from build123d import *

# Parameters (mm, degrees)
BOSS_EXTRUDE1_DEPTH = 20
SKETCH2_R           = 7.5
BOSS_EXTRUDE2_DEPTH = 85
SKETCH4_R           = 6.5
BOSS_EXTRUDE3_DEPTH = 20
SKETCH5_W           = 60
SKETCH5_H           = 10
CUT_EXTRUDE1_DEPTH  = 2
FILLET1_R           = 0.5
FILLET2_R           = 0.5


with BuildPart() as part:
    # Sketch1 → Boss-Extrude1 (new body)
    with BuildSketch(Plane.XY):
        with BuildLine():
            Line((0, 0), (0, 25.5))
            ThreePointArc((0, 25.5), (2.928932188, 32.571067812), (10, 35.5))
            Line((10, 35.5), (85, 35.5))
            ThreePointArc((85, 35.5), (92.071067812, 32.571067812), (95, 25.5))
            Line((95, 25.5), (95, -25.5))
            ThreePointArc((95, -25.5), (92.071067812, -32.571067812), (85, -35.5))
            Line((85, -35.5), (10, -35.5))
            ThreePointArc((10, -35.5), (2.928932188, -32.571067812), (0, -25.5))
            Line((0, -25.5), (0, 0))
        make_face()
        with BuildLine():
            Line((10, 0), (10, 15.5))
            ThreePointArc((10, 15.5), (12.928932188, 22.571067812), (20, 25.5))
            Line((20, 25.5), (75, 25.5))
            ThreePointArc((75, 25.5), (82.071067812, 22.571067812), (85, 15.5))
            Line((85, 15.5), (85, 0))
            Line((85, 0), (85, -15.5))
            ThreePointArc((85, -15.5), (82.071067812, -22.571067812), (75, -25.5))
            Line((75, -25.5), (20, -25.5))
            ThreePointArc((20, -25.5), (12.928932188, -22.571067812), (10, -15.5))
            Line((10, -15.5), (10, 0))
        make_face(mode=Mode.SUBTRACT)
    extrude(amount=BOSS_EXTRUDE1_DEPTH)

    # Sketch2 → Boss-Extrude2 (add)
    with BuildSketch(Plane(origin=(0, 0, 0), x_dir=(0, 0, -1), z_dir=(1, 0, 0))):
        with Locations((-10, 0)):
            Circle(SKETCH2_R)
    extrude(amount=BOSS_EXTRUDE2_DEPTH)

    # Sketch4 → Boss-Extrude3 (add)
    with BuildSketch(Plane(origin=(0, 0, 0), x_dir=(0, 0, -1), z_dir=(1, 0, 0))):
        with Locations((-10, 0)):
            Circle(SKETCH4_R)
    extrude(amount=-BOSS_EXTRUDE3_DEPTH)

    # Sketch5 → Cut-Extrude1 (cut)
    with BuildSketch(Plane.XZ.offset(35.5)):
        with Locations((48, 10.5)):
            Rectangle(SKETCH5_W, SKETCH5_H)
    cut_extrude1 = extrude(amount=-CUT_EXTRUDE1_DEPTH, mode=Mode.SUBTRACT)

    # Mirror1: Cut-Extrude1 across plane
    add(cut_extrude1.mirror(Plane.ZX), mode=Mode.SUBTRACT)

    # Fillet1
    fillet1_edges = [part.edges().sort_by_distance(p)[0] for p in [
        (47.5, 35.5, 0),
        (92.071067812, 32.571067812, 0),
        (95, 0, 0),
        (92.071067812, -32.571067812, 0),
        (47.5, -35.5, 0),
        (2.928932188, -32.571067812, 0),
        (47.5, -35.5, 20),
        (92.071067812, -32.571067812, 20),
        (95, 0, 20),
        (92.071067812, 32.571067812, 20),
        (47.5, 35.5, 20),
        (2.928932188, 32.571067812, 20),
        (0, 0, 20),
        (2.928932188, -32.571067812, 20),
        (0, 0, 0),
        (2.928932188, 32.571067812, 0),
    ]]
    fillet(fillet1_edges, radius=FILLET1_R)

    # Fillet2
    fillet2_edges = [part.edges().sort_by_distance(p)[0] for p in [
        (12.928932188, -22.571067812, 0),
        (47.5, -25.5, 0),
        (82.071067812, -22.571067812, 0),
        (85, 0, 0),
        (82.071067812, 22.571067812, 0),
        (47.5, 25.5, 0),
        (12.928932188, 22.571067812, 0),
        (10, 0, 0),
        (10, 0, 20),
        (12.928932188, -22.571067812, 20),
        (47.5, -25.5, 20),
        (82.071067812, -22.571067812, 20),
        (85, 0, 20),
        (82.071067812, 22.571067812, 20),
        (47.5, 25.5, 20),
        (12.928932188, 22.571067812, 20),
    ]]
    fillet(fillet2_edges, radius=FILLET2_R)


solid = part.part
Geometry: final body of the model. Coordinates: model frame, mm. A direction names the side the tool comes from. Give positions to 0.01 mm unless a question says otherwise; leave off trailing zeros. Write each loop counter-clockwise with the first axis right and the second up, starting at its lowest first coordinate (ties: lowest second). Pieces come first, ordered by that corner, then holes.
(1) Ray query, line 1 (Y direction, x = 46, z = 2); line 2 (Y direction, x = 72, z = 14.75); line 3 (X direction, y = -16, z = 10). Return the intervals inside material, ascending.
(2) First-contact query: P1, Ø1.6, axis at y = 34, z = 10.5, coming from the -X side; P2, Ø8, axis at x = 61, y = -22.5, coming from the -Z side; P3, Ø1.6, axis at y = 34.5, z = 8, coming from the +X side; P4, Ø2, axis at x = 23.5, z = 11, coming from the -Y side. Flat tips, straight axial feed; report the tip coordinate or a pass-through.
(3) Cut plane D-D, the plane x = -10. Return loops of the section in (y, z), then the cut area to 3 significant figures.
(4) Cut plane A-A, the plane x = 25.5. Return loops of the section in (y, z), then the cut area to 3 significant figures.
(5) Cut plane C-C, the plane y = 0. Return loops of the section in (x, z), then the cut area to 3 significant figures.
(6) Cut plane B-B, the plane z = 10. Give the number of separate pieces and of enclosed holes in the cut face, then the cut area to 4 significant figures.
(7) Access query for faces 5 (the flat face through (47, 25.5, 10)), 6 (the cylindrical face through (-9.86, 1.95, 3.8)), 7 (the flat face through (48, -35.5, 4)). Directions: +Z, -Z, +X, -X, +Y, -Y. A direction counts if a zero-diameter tool reaches every point of the face in a straight line with its end or side. Return the directions, or none.
(8) Mould query, pull axis Z, two halves, no side actions, for faces 1 (the flat face through (95, 0, 10)), 2 (the flat face through (48, -33.5, 11)), 3 (the cylindrical face through (47, 5.1, 15.5)), 4 (the flat face through (48, 33.5, 11)). Classes: released by +Z, released by -Z, zero draft, split by the parting line, or undercut.
Values follow:
1. line 1: y = -35.5 to -25.5, 25.5 to 35.5
1. line 2: y = -33.5 to -25.5, -5.8 to 5.8, 25.5 to 33.5
1. line 3: x = 0 to 10.01, 84.99 to 95
2. P1: stops at x = 3.62
2. P2: stops at z = 0
2. P3: stops at x = 90.72
2. P4: stops at y = -33.5
3. outline: circle Ø13 at (0, 10)
3. area: 133 mm2
4. outline: (-35.5, 0.5) arc R0.5 ccw to (-35, 0) - (-26, 0) arc R0.5 ccw to (-25.5, 0.5) - (-25.5, 19.5) arc R0.5 ccw to (-26, 20) - (-35, 20) arc R0.5 ccw to (-35.5, 19.5) - (-35.5, 15.5) - (-33.5, 15.5) - (-33.5, 5.5) - (-35.5, 5.5) - close; circle Ø15 at (0, 10); (25.5, 0.5) arc R0.5 ccw to (26, 0) - (35, 0) arc R0.5 ccw to (35.5, 0.5) - (35.5, 5.5) - (33.5, 5.5) - (33.5, 15.5) - (35.5, 15.5) - (35.5, 19.5) arc R0.5 ccw to (35, 20) - (26, 20) arc R0.5 ccw to (25.5, 19.5) - close
4. area: 536 mm2
5. outline: (-20, 3.5) - (0, 3.5) - (0, 0.5) arc R0.5 ccw to (0.5, 0) - (9.5, 0) arc R0.5 ccw to (10, 0.5) - (10, 2.5) - (85, 2.5) - (85, 0.5) arc R0.5 ccw to (85.5, 0) - (94.5, 0) arc R0.5 ccw to (95, 0.5) - (95, 19.5) arc R0.5 ccw to (94.5, 20) - (85.5, 20) arc R0.5 ccw to (85, 19.5) - (85, 17.5) - (10, 17.5) - (10, 19.5) arc R0.5 ccw to (9.5, 20) - (0.5, 20) arc R0.5 ccw to (0, 19.5) - (0, 16.5) - (-20, 16.5) - close
5. area: 1,780 mm2
6. separate pieces: 1
6. enclosed holes: 2
6. area: 4,065 mm2
7. face 5: +Z, -Z
7. face 6: -X
7. face 7: +Z, -Z, +X, -X, -Y
8. face 1: zero draft
8. face 2: undercut
8. face 3: split by the parting line
8. face 4: undercut
